Geometry: final body of the model. Coordinates: model frame, mm. A direction names the side the tool comes from. Round coordinates to 2 decimals unless told otherwise and drop trailing zeros. Loops run counter-clockwise (first coordinate to the right, second up) from the corner with the lowest first, then second, coordinate; pieces in that order, holes last. Notation, with made-up numbers: (-3.75, -1.75) -> (39.25, -1.75) arc R20 cw to (39.25, 8.25) -> close; hole circle Ø10 at (2, -31.5). An arc over 180 degrees is marked (long way). Answer in a Markdown table with one row per item.
```python
from build123d import *

# Parameters (mm, degrees)
SKETCH2_W                     = 75
SKETCH2_H                     = 90
BOSS_EXTRUDE1_DEPTH           = 23
SKETCH3_W                     = 18
SKETCH3_H                     = 26
CUT_EXTRUDE1_DEPTH            = 91.437823946
SKETCH4_R                     = 10
BOSS_EXTRUDE2_DEPTH           = 18
SKETCH5_R                     = 13
BOSS_EXTRUDE3_DEPTH           = 3
F_12_0_12_DIAMETER_HOLE1_D    = 12
CUT_EXTRUDE2_DEPTH            = 5
F_8_0_8_DIAMETER_HOLE1_D      = 8
M8_TAPPED_HOLE1_D             = 6.8
SKETCH17_R                    = 8
CUT_EXTRUDE3_DEPTH            = 38
F_8_0_8_DIAMETER_HOLE2_D      = 8
CHAMFER1_SIZE                 = 8
G1_8_TAPPED_HOLE1_D           = 8.8
G1_8_TAPPED_HOLE1_DEPTH       = 14
G1_8_TAPPED_HOLE1_TIP         = 2.643786724
F_2_0_2_DIAMETER_HOLE1_REACH  = 107.844
F_2_0_2_DIAMETER_HOLE1_BORE_R = 1
M6_TAPPED_HOLE1_REACH         = 107.844
M6_TAPPED_HOLE1_BORE_R        = 2.5
CIRPATTERN1_COUNT             = 4
SKETCH36_R                    = 10
CUT_EXTRUDE5_DEPTH            = 38
M8_TAPPED_HOLE2_D             = 6.8
M8_TAPPED_HOLE2_CSINK_D       = 8.05
M8_TAPPED_HOLE2_CSINK_ANGLE   = 90


with BuildPart() as part:
    # Sketch2 → Boss-Extrude1 (new, symmetric)
    with BuildSketch(Plane.XY):
        with Locations((0.5, 0)):
            Rectangle(SKETCH2_W, SKETCH2_H)
    extrude(amount=BOSS_EXTRUDE1_DEPTH, both=True)

    # Sketch3 → Cut-Extrude1 (cut, through all)
    with BuildSketch(Plane(origin=(38, 0, 0), x_dir=(0, 0, -1), z_dir=(1, 0, 0))):
        with Locations((0, -32)):
            Rectangle(SKETCH3_W, SKETCH3_H)
        with Locations((0, 32)):
            Rectangle(SKETCH3_W, SKETCH3_H)
    extrude(amount=-CUT_EXTRUDE1_DEPTH, mode=Mode.SUBTRACT)

    # Sketch4 → Boss-Extrude2 (add)
    with BuildSketch(Plane(origin=(38, 0, 0), x_dir=(0, 0, -1), z_dir=(1, 0, 0))):
        with Locations(Location((0, 0, 0), (0, 0, 180))):
            Circle(SKETCH4_R)
    extrude(amount=BOSS_EXTRUDE2_DEPTH)

    # Sketch5 → Boss-Extrude3 (add)
    with BuildSketch(Plane(origin=(38, 0, 0), x_dir=(0, 0, -1), z_dir=(1, 0, 0))):
        with Locations(Location((0, 0, 0), (0, 0, 180))):
            Circle(SKETCH5_R)
    extrude(amount=BOSS_EXTRUDE3_DEPTH)

    # Ø12.0 (12) Diameter Hole1 (through all)
    with Locations(Plane(origin=(0, 0, -23), x_dir=(-1, 0, 0), z_dir=(0, 0, -1))):
        with Locations((0, 0)):
            Hole(F_12_0_12_DIAMETER_HOLE1_D / 2)

    # Sketch9 → Cut-Extrude2 (cut)
    with BuildSketch(Plane(origin=(0, 0, -23), x_dir=(-1, 0, 0), z_dir=(0, 0, -1))):
        with BuildLine():
            Line((-9.5, -45), (-9.5, -36))
            ThreePointArc((-9.5, -36), (-0.5, -27), (8.5, -36))
            Line((8.5, -36), (8.5, -45))
            ThreePointArc((8.5, -45), (-0.5, -54), (-9.5, -45))
        make_face()
        with BuildLine():
            Line((-9.5, 45), (-9.5, 36))
            ThreePointArc((-9.5, 36), (-0.5, 27), (8.5, 36))
            Line((8.5, 36), (8.5, 45))
            ThreePointArc((8.5, 45), (-0.5, 54), (-9.5, 45))
        make_face()
    cut_extrude2 = extrude(amount=-CUT_EXTRUDE2_DEPTH, mode=Mode.SUBTRACT)

    # Mirror1: Cut-Extrude2 across plane
    add(cut_extrude2.mirror(Plane.XY), mode=Mode.SUBTRACT)

    # Ø8.0 (8) Diameter Hole1 (through all)
    with Locations(Plane(origin=(0, 0, -18), x_dir=(-1, 0, 0), z_dir=(0, 0, -1))):
        with Locations((-0.5, -36), (-0.5, 36)):
            Hole(F_8_0_8_DIAMETER_HOLE1_D / 2)

    # M8 Tapped Hole1 (through all)
    with Locations(Plane(origin=(0, 0, -23), x_dir=(-1, 0, 0), z_dir=(0, 0, -1))):
        with Locations((0, 13.5), (0, -13.5)):
            Hole(M8_TAPPED_HOLE1_D / 2)

    # Sketch17 → Cut-Extrude3 (cut)
    with BuildSketch(Plane(origin=(0, 45, 0), x_dir=(1, 0, 0), z_dir=(0, 1, 0))):
        with Locations(Location((24, 0, 0), (0, 0, 180))):
            Circle(SKETCH17_R)
    cut_extrude3 = extrude(amount=-CUT_EXTRUDE3_DEPTH, mode=Mode.SUBTRACT)

    # Mirror2: Cut-Extrude3 across plane
    add(cut_extrude3.mirror(Plane.ZX), mode=Mode.SUBTRACT)

    # Ø8.0 (8) Diameter Hole2 (through all)
    with Locations(Plane(origin=(0, 7, 0), x_dir=(1, 0, 0), z_dir=(0, 1, 0))):
        with Locations((24, 0)):
            Hole(F_8_0_8_DIAMETER_HOLE2_D / 2)

    # Chamfer1
    chamfer1_edges = [part.edges().sort_by_distance(p)[0] for p in [
        (-37, 45, -16),
        (-37, -45, -16),
        (-37, 45, 16),
        (-37, -45, 16),
    ]]
    chamfer(chamfer1_edges, length=CHAMFER1_SIZE)

    # G1/8 Tapped Hole1
    with Locations(Plane(origin=(56, 0, 0), x_dir=(0, 0, -1), z_dir=(1, 0, 0))):
        with Locations((0, 0)):
            Hole(G1_8_TAPPED_HOLE1_D / 2, depth=G1_8_TAPPED_HOLE1_DEPTH)
            with Locations((0, 0, -(G1_8_TAPPED_HOLE1_DEPTH + G1_8_TAPPED_HOLE1_TIP / 2))):  # 118° drill point
                Cone(0, G1_8_TAPPED_HOLE1_D / 2, G1_8_TAPPED_HOLE1_TIP, mode=Mode.SUBTRACT)

    # Ø2.0 (2) Diameter Hole1 bore → Ø2.0 (2) Diameter Hole1 (cut, up to next)
    with BuildSketch(Plane(origin=(56, 0, 0), x_dir=(0, 0, -1), z_dir=(1, 0, 0)), mode=Mode.PRIVATE) as f_2_0_2_diameter_hole1_sk1:
        Circle(F_2_0_2_DIAMETER_HOLE1_BORE_R)
    f_2_0_2_diameter_hole1_tool1 = extrude(f_2_0_2_diameter_hole1_sk1.sketch, amount=-F_2_0_2_DIAMETER_HOLE1_REACH, mode=Mode.PRIVATE) & part.part
    add(f_2_0_2_diameter_hole1_tool1.solids().sort_by_distance((56, 0, 0))[0], mode=Mode.SUBTRACT)

    # M6 Tapped Hole1 bore → M6 Tapped Hole1 (cut, up to next)
    with BuildSketch(Plane.ZY.offset(37), mode=Mode.PRIVATE) as m6_tapped_hole1_sk1:
        Circle(M6_TAPPED_HOLE1_BORE_R)
    m6_tapped_hole1_tool1 = extrude(m6_tapped_hole1_sk1.sketch, amount=-M6_TAPPED_HOLE1_REACH, mode=Mode.PRIVATE) & part.part
    add(m6_tapped_hole1_tool1.solids().sort_by_distance((-37, 0, 0))[0], mode=Mode.SUBTRACT)

    # Sketch34 → M6 Tapped Hole2 (revolve, cut)
    with BuildSketch(Plane(origin=(38, 16.263455967, 16.263455967), x_dir=(0, 0, -1), z_dir=(0, 1, 0))):
        Polygon((0, 0), (0, 16.502151548), (2.5, 15), (2.5, 0), align=None)
    m6_tapped_hole2 = revolve(axis=Axis((44.35, 16.263455967, 16.263455967), (-1, 0, 0)), mode=Mode.SUBTRACT)

    # CirPattern1: M6 Tapped Hole2 ×4 about axis
    cirpattern1_axis = Axis((0, 0, 0), (1, 0, 0))
    for i in range(1, CIRPATTERN1_COUNT):
        add(m6_tapped_hole2.rotate(cirpattern1_axis, i * 360 / CIRPATTERN1_COUNT), mode=Mode.SUBTRACT)

    # Sketch36 → Cut-Extrude5 (cut)
    with BuildSketch(Plane.XZ.offset(45)):
        with Locations((-22, 0)):
            Circle(SKETCH36_R)
    cut_extrude5 = extrude(amount=-CUT_EXTRUDE5_DEPTH, mode=Mode.SUBTRACT)

    # Mirror4: Cut-Extrude5 across plane
    add(cut_extrude5.mirror(Plane.ZX), mode=Mode.SUBTRACT)

    # M8 Tapped Hole2 (through all)
    with Locations(Plane(origin=(0, -7, 0), x_dir=(-1, 0, 0), z_dir=(0, -1, 0))):
        with Locations((22, 0)):
            CounterSinkHole(M8_TAPPED_HOLE2_D / 2, M8_TAPPED_HOLE2_CSINK_D / 2, counter_sink_angle=M8_TAPPED_HOLE2_CSINK_ANGLE)


solid = part.part
```
Item 1: Section query B-B, the plane y = 24. Output: boundary loops of the cut face in (x, z).
Ans:
| item | result |
|---|---|
| outline | (-37, -23) -> (38, -23) -> (38, -9) -> (-17.64, -9) arc R10 cw to (-26.36, -9) -> (-37, -9) -> close; (-37, 9) -> (-26.36, 9) arc R10 cw to (-17.64, 9) -> (38, 9) -> (38, 23) -> (-37, 23) -> close |
Item 2: First-contact query: P1, Ø6, axis at x = -26, z = 0, coming from the +Y side; P2, Ø3, axis at y = 10.5, z = -12, coming from the +X side; P3, Ø2.5, axis at y = -42.5, z = -20, coming from the -X side. Flat tips, straight axial feed; report the tip coordinate or a pass-through.
Ans:
| item | result |
|---|---|
| P1 | y = 7 |
| P2 | x = 38 |
| P3 | x = -32.75 |
Item 3: Section query A-A, the plane x = -22. Output: boundary loops of the cut face in (y, z) (3 decimals), and give its area (3 significant figures).
Ans:
| item | result |
|---|---|
| outline | (-45, -23) -> (45, -23) -> (45, -10) -> (7, -10) -> (7, -3.4) -> (-6.375, -3.4) -> (-7, -4.025) -> (-7, -10) -> (-45, -10) -> close; (-45, 10) -> (-7, 10) -> (-7, 4.025) -> (-6.375, 3.4) -> (7, 3.4) -> (7, 10) -> (45, 10) -> (45, 23) -> (-45, 23) -> close |
| area | 2,520 mm2 |
Item 4: Ray query, L1, parallel to Y at x = 0, z = -5.5; L2, parallel to Y at x = -30.5, z = 0; L3, parallel to Z at x = 24, y = 3. Return the intervals inside material, ascending.
Ans:
| item | result |
|---|---|
| L1 | -19 to -16.9, -10.1 to -6, 6 to 10.1, 16.9 to 19 |
| L2 | -7 to -2.5, 2.5 to 7 |
| L3 | -23 to -4, 4 to 23 |
Item 5: Section query D-D, the plane x = 0. State how many separate pieces and enclosed holes the cut face has, and give its area (3 significant figures).
Ans:
| item | result |
|---|---|
| separate pieces | 8 |
| enclosed holes | 0 |
| area | 1,380 mm2 |
Item 6: Section query C-C, the plane x = 29.5. Output: boundary loops of the cut face in (y, z).
Ans:
| item | result |
|---|---|
| outline | (-45, -23) -> (45, -23) -> (45, -9) -> (19, -9) -> (19, -5.81) -> (7, -5.81) -> (7, 5.81) -> (19, 5.81) -> (19, 9) -> (45, 9) -> (45, 23) -> (-45, 23) -> (-45, 9) -> (-19, 9) -> (-19, 5.81) -> (-7, 5.81) -> (-7, -5.81) -> (-19, -5.81) -> (-19, -9) -> (-45, -9) -> close; hole circle Ø5 at (-16.26, -16.26); hole circle Ø5 at (-16.26, 16.26); hole circle Ø2 at (0, 0); hole circle Ø5 at (16.26, -16.26); hole circle Ø5 at (16.26, 16.26) |
Item 7: Mould query, pull axis Y, two halves, no side actions, for faces 5 (the conical face through (21.759, 16.03, -15.897)), 6 (the cylindrical face through (0.698, 27.002, -20.535)), 7 (the cylindrical face through (-0.74, 10.18, 0.32)), 8 (the flat face through (-8.5, -40, -21)). Classes: released by +Y, released by -Y, zero draft, split by the parting line, or undercut.
Ans:
| item | result |
|---|---|
| face 5 | undercut |
| face 6 | released by +Y |
| face 7 | undercut |
| face 8 | zero draft |
Item 8: Set-up query: faces 1 (the cylindrical face through (39.479, 7.91, -10.316)), 2 (the flat face through (-8.5, -40, 21)), 3 (the flat face through (-1, 40, 18)), 4 (the flat face through (-32, -32, -9)). Return all of +Z, -Z, +X, -X, +Y, -Y with unobstructed straight access to the full face (end or side cutting, diameter ignored); none if empty.
Ans:
| item | result |
|---|---|
| face 1 | +X |
| face 2 | +Z, -Y |
| face 3 | +Z, +Y |
| face 4 | +X, -X, -Y |
